For this review, use the dimensioned drawing (mm, ordinates from the lowest corner) and the shaded views. Coordinates: 2 decimals unless noted, no trailing zeros. Order: outer loops, then holes, each group sorted by start corner. A loop starts at its lowest first (then second) coordinate and runs counter-clockwise, first axis right, second up. Notation, with made-up numbers: (8, 18) -> (57, 18) arc R25 cw to (57, 36) -> close; hole circle Ø11 at (60, -5.5). An arc over 180 degrees is marked (long way). Use one line per item in the form item = value. Start each with the question number.
(1) Insertion check: pin 1 Ø6 at (x, z) = (56, 11) entering from +Y (3 decimals); pin 2 Ø11 at (x, y) = (40, 12.5) entering from -Z (3 decimals). Each pin has a flat end and moves straight along its axis. Give the tip position at first contact, or say it passes through.
(2) Wall thickness on line 1 along Y through (x, z) = (93, 10) (3 decimals); line 2 along Z through (x, y) = (45.5, 11.5) (3 decimals); line 3 along Y through (x, z) = (70, 23.5) (1 decimal): over which ranges is each line inside the solid? List them lowest first.
(3) Take a section at D-D (y = 5.75). State the section outline as (x, z) points (3 decimals).
(4) Take a section at B-B (y = 20.5). State the section outline as (x, z) points (1 decimal).
(5) Mouldability with a two-part tool opening along Y and no side actions: class the marked faces 1, 2 and 3 as +Y half, -Y half, draft (parallel to the pull), parting line (faces both ways), or undercut.
(6) Take a section at C-C (x = 107). State the section outline as (y, z) points (3 decimals), then the cut area to 3 significant figures.
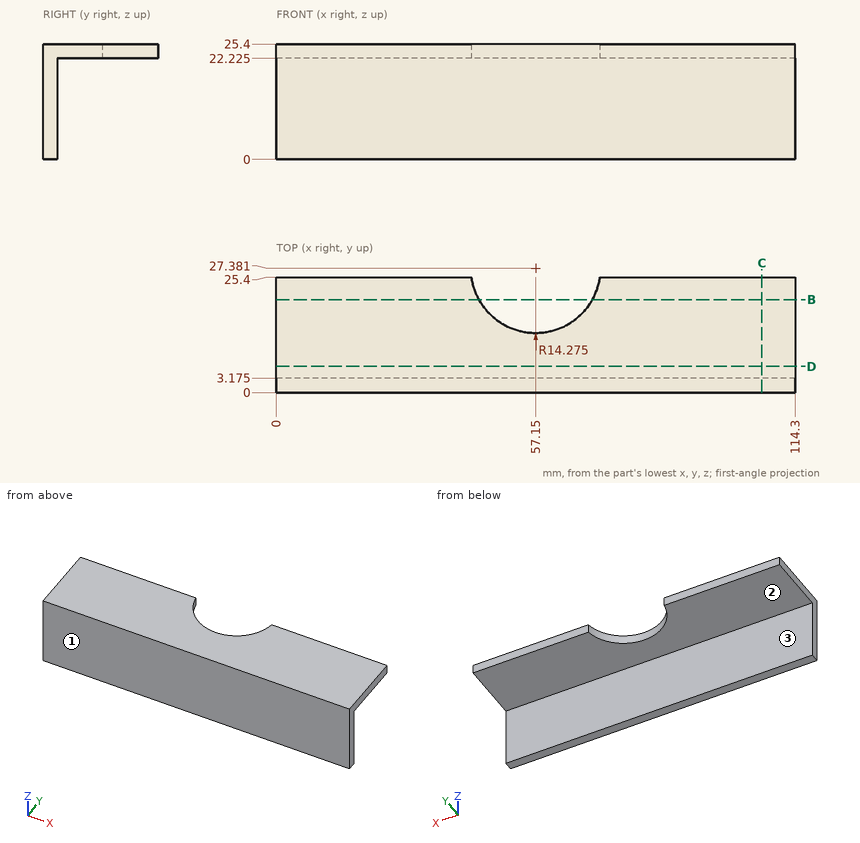
Findings:
q1.pin_1 = 3.175
q1.pin_2 = 22.225
q2.line_1 = 0 to 3.175
q2.line_2 = 22.225 to 25.4
q2.line_3 = 0 to 21.2
q3.outline = (0, 22.225) -> (114.3, 22.225) -> (114.3, 25.4) -> (0, 25.4) -> close
q4.outline = (0, 22.2) -> (44.6, 22.2) -> (44.6, 25.4) -> (0, 25.4) -> close; (69.7, 22.2) -> (114.3, 22.2) -> (114.3, 25.4) -> (69.7, 25.4) -> close
q5.face_1 = -Y half
q5.face_2 = draft
q5.face_3 = +Y half
q6.outline = (0, 0) -> (3.175, 0) -> (3.175, 22.225) -> (25.4, 22.225) -> (25.4, 25.4) -> (0, 25.4) -> close
q6.area = 151 mm²
